Could you check a few things on this model? Use its own coordinates, in mm. Face numbers are marked on the shaded views. A direction names the side the tool comes from. Give positions to 0.01 mm unless a question says otherwise; leave off trailing zeros. Order: outer loops, then holes, each group sorted by start corner. A loop starts at its lowest first (then second) coordinate and runs counter-clockwise, first axis right, second up.
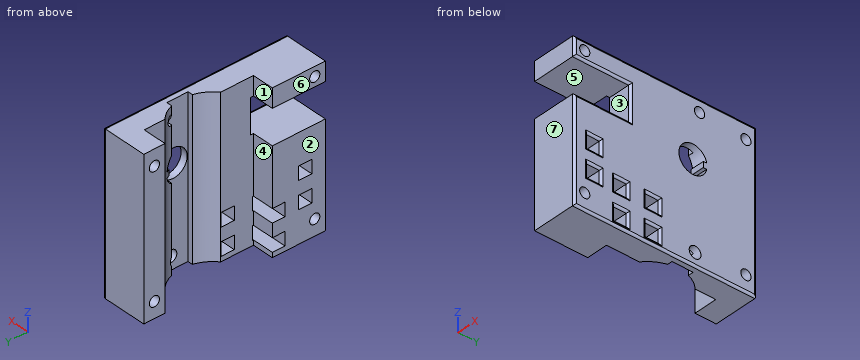
from build123d import *

# Parameters (mm, degrees)
PROFILEEXTRUDE_DEPTH = 73.76
HOSEWINDOW_W         = 16.29
HOSEWINDOW_H         = 26.5
HOSEWINDOWCUT_DEPTH  = 22.63
CAGESCREWS_R         = 2.4
CAGESCREWSCUT_DEPTH  = 22.63
AXLEHOLECUT_DEPTH    = 22.63
SETSCREWS_R          = 2.426338021
SETSCREWS_R_2        = 2.788762315
SETSCREWSCUT_DEPTH   = 22.63
SKETCH1_W            = 6.35
SKETCH1_H            = 6.35
CUT_EXTRUDE1_DEPTH   = 22.63
FILLET1_R            = 1


with BuildPart() as part:
    # Profile → ProfileExtrude (new body)
    with BuildSketch(Plane.XY):
        with BuildLine():
            Line((-6.01073477, -58.62791746), (-6.01073477, -33.62791746))
            Line((-6.01073477, -33.62791746), (4.13926523, -33.62791746))
            Line((4.13926523, -33.62791746), (4.13926523, -18.13791746))
            ThreePointArc((4.13926523, -18.13791746), (7.563334043, -14.326029686), (9.63126523, -9.63791746))
            Line((9.63126523, -9.63791746), (11.94926523, -9.63791746))
            Line((11.94926523, -9.63791746), (11.94926523, 0.36208254))
            Line((11.94926523, 0.36208254), (9.35926523, 0.36208254))
            ThreePointArc((9.35926523, 0.36208254), (7.525939238, 4.313848402), (4.70926523, 7.63708254))
            Line((4.70926523, 7.63708254), (4.70926523, 17.41208254))
            Line((4.70926523, 17.41208254), (-6.44073477, 17.41208254))
            Line((-6.44073477, 17.41208254), (-6.44073477, 27.41208254))
            Line((-6.44073477, 27.41208254), (15.18926523, 27.41208254))
            Line((15.18926523, 27.41208254), (15.18926523, -58.62791746))
            Line((15.18926523, -58.62791746), (-6.01073477, -58.62791746))
        make_face()
    extrude(amount=PROFILEEXTRUDE_DEPTH)

    # HoseWindow → HoseWindowCut (cut, through all)
    with BuildSketch(Plane(origin=(15.18926523, 0, 0), x_dir=(0, 0, -1), z_dir=(1, 0, 0))):
        with Locations((-56.725, -45.37791746)):
            Rectangle(HOSEWINDOW_W, HOSEWINDOW_H)
    extrude(amount=-HOSEWINDOWCUT_DEPTH, mode=Mode.SUBTRACT)

    # CageScrews → CageScrewsCut (cut, through all)
    with BuildSketch(Plane(origin=(15.18926523, 0, 0), x_dir=(0, 0, -1), z_dir=(1, 0, 0))):
        with Locations((-66.26, 22.41208254)):
            Circle(CAGESCREWS_R)
        with Locations((-7.5, 22.41208254)):
            Circle(CAGESCREWS_R)
        with Locations((-7.5, -53.62791746)):
            Circle(CAGESCREWS_R)
        with Locations((-69.31, -53.62791746)):
            Circle(CAGESCREWS_R)
    extrude(amount=-CAGESCREWSCUT_DEPTH, mode=Mode.SUBTRACT)

    # AxleHole → AxleHoleCut (cut, through all)
    with BuildSketch(Plane(origin=(15.18926523, 0, 0), x_dir=(0, 0, -1), z_dir=(1, 0, 0))):
        with BuildLine():
            Line((-44.699, 2.307293484), (-47.361, 2.307293484))
            Line((-47.361, 2.307293484), (-47.361, 3.926293484))
            ThreePointArc((-47.361, 3.926293484), (-46.03, -9.21691746), (-44.699, 3.926293484))
            Line((-44.699, 3.926293484), (-44.699, 2.307293484))
        make_face()
    extrude(amount=-AXLEHOLECUT_DEPTH, mode=Mode.SUBTRACT)

    # SetScrews → SetScrewsCut (cut, through all)
    with BuildSketch(Plane(origin=(15.18926523, 0, 0), x_dir=(0, 0, -1), z_dir=(1, 0, 0))):
        with Locations((-67.80722939, 0.544946624)):
            Circle(SETSCREWS_R)
        with Locations((-6.04299884, -1.55824191)):
            Circle(SETSCREWS_R_2)
    extrude(amount=-SETSCREWSCUT_DEPTH, mode=Mode.SUBTRACT)

    # Sketch1 → Cut-Extrude1 (cut, through all)
    with BuildSketch(Plane(origin=(15.18926523, 0, 0), x_dir=(0, 0, -1), z_dir=(1, 0, 0))):
        with Locations((-18.175, -49.10291746)):
            Rectangle(SKETCH1_W, SKETCH1_H)
        with Locations((-30.875, -49.10291746)):
            Rectangle(SKETCH1_W, SKETCH1_H)
        with Locations((-5.475, -36.40291746)):
            Rectangle(SKETCH1_W, SKETCH1_H)
        with Locations((-18.175, -36.40291746)):
            Rectangle(SKETCH1_W, SKETCH1_H)
        with Locations((-5.475, -21.40291746)):
            Rectangle(SKETCH1_W, SKETCH1_H)
        with Locations((-18.175, -21.40291746)):
            Rectangle(SKETCH1_W, SKETCH1_H)
    extrude(amount=-CUT_EXTRUDE1_DEPTH, mode=Mode.SUBTRACT)

    # Fillet1
    fillet1_edges = [part.edges().sort_by_distance(p)[0] for p in [
        (15.18926523, -45.92791746, 18.175),
        (15.18926523, -49.10291746, 21.35),
        (15.18926523, -52.27791746, 18.175),
        (15.18926523, -49.10291746, 15),
        (15.18926523, -45.92791746, 30.875),
        (15.18926523, -49.10291746, 34.05),
        (15.18926523, -52.27791746, 30.875),
        (15.18926523, -49.10291746, 27.7),
        (15.18926523, -33.22791746, 5.475),
        (15.18926523, -36.40291746, 8.65),
        (15.18926523, -39.57791746, 5.475),
        (15.18926523, -36.40291746, 2.3),
        (15.18926523, -15.60791746, 0),
        (15.18926523, -33.22791746, 18.175),
        (15.18926523, -36.40291746, 21.35),
        (15.18926523, -39.57791746, 18.175),
        (15.18926523, -36.40291746, 15),
        (15.18926523, -18.22791746, 5.475),
        (15.18926523, -21.40291746, 8.65),
        (15.18926523, -24.57791746, 5.475),
        (15.18926523, -21.40291746, 2.3),
        (15.18926523, -18.22791746, 18.175),
        (15.18926523, -21.40291746, 21.35),
        (15.18926523, -24.57791746, 18.175),
        (15.18926523, -21.40291746, 15),
        (15.18926523, -58.62791746, 69.315),
        (15.18926523, 27.41208254, 36.88),
        (15.18926523, -58.62791746, 24.29),
        (15.18926523, -15.60791746, 73.76),
        (15.18926523, -45.37791746, 64.87),
        (15.18926523, -45.37791746, 48.58),
        (15.18926523, -32.12791746, 56.725),
    ]]
    fillet(fillet1_edges, radius=FILLET1_R)


solid = part.part
Item 1: Imagine slicing it at B-B on y = -44. List the corners of the cut face in (x, z) for me.
Findings:
outline: (-6.01, 0) - (14.19, 0) arc R1 ccw to (15.19, 1) - (15.19, 47.58) arc R1 ccw to (14.19, 48.58) - (-6.01, 48.58) - close; (-6.01, 64.87) - (14.19, 64.87) arc R1 ccw to (15.19, 65.87) - (15.19, 72.76) arc R1 ccw to (14.19, 73.76) - (-6.01, 73.76) - close
Item 2: Imagine slicing it at D-D on z = 36.5. List the corners of the cut face in (x, y) for me.
Findings:
outline: (-6.44, 17.41) - (4.71, 17.41) - (4.71, 7.64) arc R16.26 cw to (9.36, 0.36) - (11.95, 0.36) - (11.95, -9.64) - (9.63, -9.64) arc R16.26 cw to (4.14, -18.14) - (4.14, -33.63) - (-6.01, -33.63) - (-6.01, -58.63) - (14.19, -58.63) arc R1 ccw to (15.19, -57.63) - (15.19, 26.41) arc R1 ccw to (14.19, 27.41) - (-6.44, 27.41) - close
Item 3: For the marked faces 4, 5, 6 and 7, which set-ups out of +Z, -Z, +X, -X, +Y, -Y let a thin tool reach every point of the face, with its end or its side?
Findings:
face 4: +Z, -Z, -X
face 5: +X, -X, -Y
face 6: +Z, -Z, -X, -Y
face 7: +Z, -Z, +X, -X, -Y
Item 4: Imagine slicing it at C-C on x = -1.5. Give the number of separate pieces and of enclosed holes in the cut face, then the cut area to 3 significant figures.
Findings:
separate pieces: 3
enclosed holes: 6
area: 1,950 mm2
Item 5: Imagine slicing it at A-A on z = 46.03. List the corners of the cut face in (x, y) for me, then the cut area to 3 significant figures.
Findings:
outline: (-6.44, 17.41) - (4.71, 17.41) - (4.71, 7.64) arc R16.26 cw to (8.62, 2.31) - (15.19, 2.31) - (15.19, 26.41) arc R1 ccw to (14.19, 27.41) - (-6.44, 27.41) - close; (-6.01, -58.63) - (14.19, -58.63) arc R1 ccw to (15.19, -57.63) - (15.19, -9.22) - (11.95, -9.22) - (11.95, -9.64) - (9.63, -9.64) arc R16.26 cw to (4.14, -18.14) - (4.14, -33.63) - (-6.01, -33.63) - close
area: 1,130 mm2
Item 6: We'd pull the mould along Y, two halves only. Please class the marked faces 1, 2 and 3: +Y half, -Y half, draft (parallel to the pull), parting line (faces both ways), or undercut.
Findings:
face 1: undercut
face 2: draft
face 3: -Y half
Item 7: Please list where these lines run through material, in increasing order: line 1 along Y through (x, z) = (3.75, 33); line 2 along Z through (x, y) = (9.5, -19); line 3 along Y through (x, z) = (1, 7.5).
Findings:
line 1: y = -58.63 to -52.28, -45.93 to -33.63, 17.41 to 27.41
line 2: z = 0 to 2.3, 8.65 to 15, 21.35 to 73.76
line 3: y = -58.63 to -56.03, -51.23 to -39.58, 17.41 to 20.01, 24.81 to 27.41
Item 8: For pin 1 (7.5 mm diameter, centred on y = -44, z = 21, fed in from -X); pin 2 (4.5 mm diameter, centred on y = -53.63, z = 7.5, fed in from +X); pin 3 (17.5 mm diameter, centred on y = -2.58, z = 46.03, fed in from -X), each with a flat end and sliding along its axis, tell me the tip position at first contact or that it passes through.
Findings:
pin 1: stops at x = -6.01
pin 2: passes through
pin 3: stops at x = 6.14
